The figure shows three views and two pictorial views of one solid part (mm, origin at its lowest corner). Answer the questions. A direction names the side the tool comes from. Coordinates: 2 decimals unless noted, no trailing zeros. Order: outer loops, then holes, each group sorted by start corner. A loop starts at its lowest first (then second) coordinate and runs counter-clockwise, first axis right, second up. Notation, with made-up numbers: (87, 61.25) -> (127, 61.25) arc R23 ccw to (127, 95.25) -> close; hole circle Ø6 at (-39.5, 44). An arc over 180 degrees is marked (long way). Write item = value, one per line.
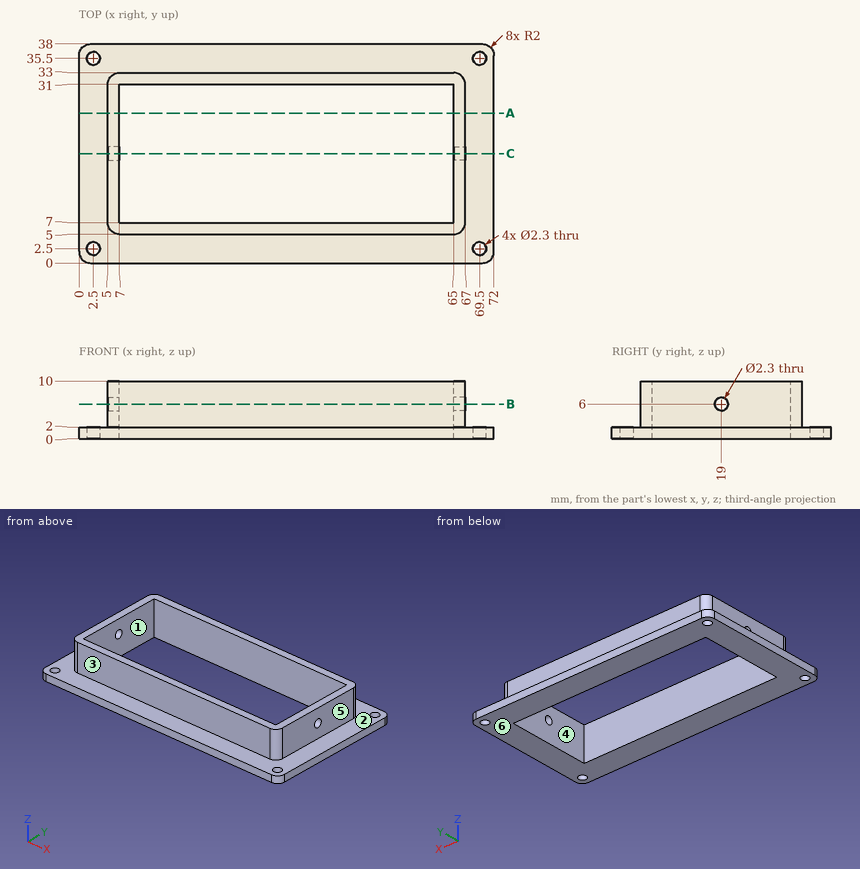
Q1. A tool of negligible diameter and unlimited length cuts with its end or side. For the marked faces 4, 5 and 6, from which of +Z, -Z, +X, -X, +Y, -Y can it reach the whole face along a straight path? Write none if from no direction.
The answers:
face_4 = +Z, -Z
face_5 = +Z, +X, +Y, -Y
face_6 = -Z, +X, -X, +Y, -Y
Q2. Find the intervals of material crossed by line 1 along X through (y, z) = (2.5, 1.5); line 2 along Y through (x, z) = (2.5, 1.25); line 3 along Y through (x, z) = (29, 1.5), in increasing order.
The answers:
line_1 = 0 to 1.35, 3.65 to 68.35, 70.65 to 72
line_2 = 0 to 1.35, 3.65 to 34.35, 36.65 to 38
line_3 = 0 to 7, 31 to 38
Q3. The mould has two halves that part along Y. Classify the marked faces 1, 2 and 3: released by +Y, released by -Y, zero draft, split by the parting line, or undercut.
The answers:
face_1 = undercut
face_2 = zero draft
face_3 = released by -Y
Q4. Section C-C, the plane y = 19 is taken. Give the vertices of the cut face in (x, z), plus the area to 3 significant figures.
The answers:
outline = (0, 0) -> (7, 0) -> (7, 4.85) -> (5, 4.85) -> (5, 2) -> (0, 2) -> close; (5, 7.15) -> (7, 7.15) -> (7, 10) -> (5, 10) -> close; (65, 0) -> (72, 0) -> (72, 2) -> (67, 2) -> (67, 4.85) -> (65, 4.85) -> close; (65, 7.15) -> (67, 7.15) -> (67, 10) -> (65, 10) -> close
area = 50.8 mm2
Q5. Section A-A, the plane y = 26 is taken. Give the vertices of the cut face in (x, z).
The answers:
outline = (0, 0) -> (7, 0) -> (7, 10) -> (5, 10) -> (5, 2) -> (0, 2) -> close; (65, 0) -> (72, 0) -> (72, 2) -> (67, 2) -> (67, 10) -> (65, 10) -> close
Q6. Each of these flat-tipped pins is pushed along its axis until it touches: pin 1 Ø2 at (x, y) = (69.5, 2.5) entering from +Z; pin 2 Ø3 at (y, z) = (18, 8) entering from -X; pin 3 Ø2.5 at (x, y) = (2.5, 35.5) entering from +Z; pin 4 Ø5 at (x, z) = (13, 7) entering from -Y. Where does it stop, or does it pass through?
The answers:
pin_1 = through
pin_2 = 5
pin_3 = 2
pin_4 = 5
Q7. Section B-B, the plane z = 6 is taken. Give the vertices of the cut face in (x, y).
The answers:
outline = (5, 7) arc R2 ccw to (7, 5) -> (65, 5) arc R2 ccw to (67, 7) -> (67, 17.85) -> (65, 17.85) -> (65, 7) -> (7, 7) -> (7, 17.85) -> (5, 17.85) -> close; (5, 20.15) -> (7, 20.15) -> (7, 31) -> (65, 31) -> (65, 20.15) -> (67, 20.15) -> (67, 31) arc R2 ccw to (65, 33) -> (7, 33) arc R2 ccw to (5, 31) -> close
